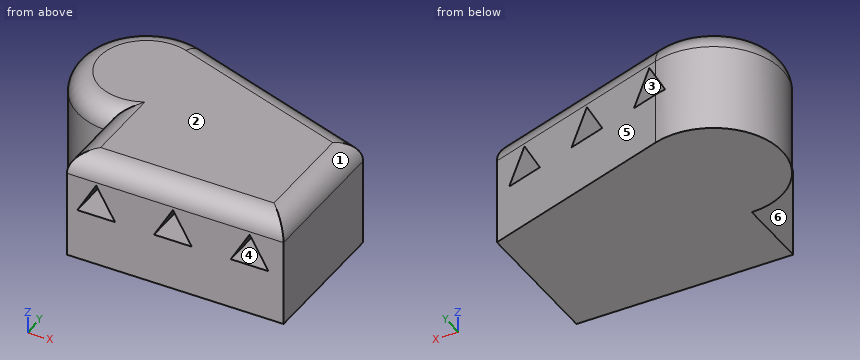
from build123d import *

# Parameters (mm, degrees)
F1_DEPTH = 25
F4_DEPTH = 25
F5_DEPTH = 23.7095438224
F6_R     = 5


# Not quite as in the source:
# - the program builds the solid bodies; features that only make, move or delete a surface that nothing else refers to are left out


with BuildPart() as f1:
    # F0 (on Top) → F1 (new body)
    with BuildSketch(Plane.XY):
        with BuildLine():
            ThreePointArc((-24.4463197887, 8.4633977604), (-29.1204506303, 19.7477478306), (-17.8361005601, 15.073616989))
            Line((-17.8361005601, 15.073616989), (-8.6304908186, 15.073616989))
            ThreePointArc((-8.6304908186, 15.073616989), (-11.6154192696, 24.3206942504), (-19.4435108685, 30.0773614855))
            ThreePointArc((-19.4435108685, 30.0773614855), (-40.0578075922, 17.607762717), (-24.4463197887, -0.7422119811))
            Line((-24.4463197887, -0.7422119811), (-24.4463197887, 8.4633977604))
        make_face()
        with BuildLine():
            Line((-17.8361005601, 15.073616989), (-24.4463197887, 15.073616989))
            Line((-24.4463197887, 15.073616989), (-24.4463197887, 8.4633977604))
            ThreePointArc((-24.4463197887, 8.4633977604), (-19.772188947, 10.3994861473), (-17.8361005601, 15.073616989))
        make_face()
        with BuildLine():
            Line((-24.4463197887, 8.4633977604), (-24.4463197887, 15.073616989))
            Line((-24.4463197887, 15.073616989), (-17.8361005601, 15.073616989))
            ThreePointArc((-17.8361005601, 15.073616989), (-29.1204506303, 19.7477478306), (-24.4463197887, 8.4633977604))
        make_face()
        with BuildLine():
            ThreePointArc((-19.4435108685, 30.0773614855), (-11.6154192696, 24.3206942504), (-8.6304908186, 15.073616989))
            Line((-8.6304908186, 15.073616989), (25.5536802113, 15.073616989))
            Line((25.5536802113, 15.073616989), (-19.4435108685, 30.0773614855))
        make_face()
        with BuildLine():
            Line((25.5536802113, 15.073616989), (-8.6304908186, 15.073616989))
            ThreePointArc((-8.6304908186, 15.073616989), (-13.2628398739, 3.8901370741), (-24.4463197887, -0.7422119811))
            Line((-24.4463197887, -0.7422119811), (-24.4463197887, -17.8190978634))
            Line((-24.4463197887, -17.8190978634), (25.5536802113, -17.8190978634))
            Line((25.5536802113, -17.8190978634), (25.5536802113, 15.073616989))
        make_face()
        with BuildLine():
            Line((-8.6304908186, 15.073616989), (-17.8361005601, 15.073616989))
            ThreePointArc((-17.8361005601, 15.073616989), (-19.772188947, 10.3994861473), (-24.4463197887, 8.4633977604))
            Line((-24.4463197887, 8.4633977604), (-24.4463197887, -0.7422119811))
            ThreePointArc((-24.4463197887, -0.7422119811), (-13.2628398739, 3.8901370741), (-8.6304908186, 15.073616989))
        make_face()
    extrude(amount=F1_DEPTH)

    # F3 (on face) → F4 (cut)
    with BuildSketch(Plane.XZ.offset(17.8190978634)):
        Polygon((-22.0338956294, 11.7883440107), (-13.3311382654, 11.7883440107), (-17.6825169474, 19.3251529709), align=None)
        Polygon((4.3688617346, 11.7883440107), (0.0174830526, 19.3251529709), (-4.3338956294, 11.7883440107), align=None)
        Polygon((22.0688617346, 11.7883440107), (17.7174830526, 19.3251529709), (13.3661043706, 11.7883440107), align=None)
    extrude(amount=-F4_DEPTH, mode=Mode.SUBTRACT)

    # F5 (cut, through all): faces of the model
    f5_faces = [f1.faces().sort_by_distance(p)[0] for p in [
        (-17.6825169474, 7.1809021366, 14.3006136641),
        (0.0174830526, 7.1809021366, 14.3006136641),
        (17.7174830526, 7.1809021366, 14.3006136641),
    ]]
    extrude(f5_faces, amount=-F5_DEPTH, mode=Mode.SUBTRACT)

    # F6
    f6_edges = [f1.edges().sort_by_distance(p)[0] for p in [
        (-40.057808, 17.607763, 25),
        (-24.44632, -9.280655, 25),
        (0.55368, -17.819098, 25),
        (25.55368, -1.37274, 25),
        (3.055085, 22.575489, 25),
    ]]
    fillet(f6_edges, radius=F6_R)


solid = f1.part
CAD build for the part. Positions are in the model's coordinates, mm. Face numbers are marked on the shaded views. A direction names the side the tool comes from. Round coordinates to 2 decimals unless told otherwise and drop trailing zeros. Write each loop counter-clockwise with the first axis right and the second up, starting at its lowest first coordinate (ties: lowest second). Pieces come first, ordered by that corner, then holes.
(1) Slice it at D-D, the plane y = 17. Count the separate pieces of the cut face and the enclosed holes in it, and give its area (3 significant figures).
(2) Slice it at A-A, the plane y = -10. Write the cut outline in (x, z).
(3) Slice it at B-B, the plane z = 17.5. Write the cut outline in (x, y), and give its area (3 significant figures).
(4) Drop flat-ended pins along their axis: P1, Ø1.5, axis at y = -4.5, z = 20.5, coming from the -X side; P2, Ø12, axis at y = 0, z = 22, coming from the -X side; P3, Ø6, axis at x = 11.5, y = 25, coming from the -Z side. Give the stop position or say it passes through.
(5) Slice it at C-C, the plane z = 11. Write the cut outline in (x, y).
(6) Probe line 1 along X through (y, z) = (-9.5, 13.25); line 2 along X through (y, z) = (17, 15.25); line 3 along X through (y, z) = (-5.5, 13.5). List the from-to ranges inside material, lowest first.
(7) Mould opens along X. For the marked faces 1, 2 and 3 say: pulls with the +X half, pulls with the -X half, needs draft (parallel to the pull), parting line crosses it, or undercut.
(8) 3-axis set-ups, long thin cutter, end or side, ignore diameter. For the marked faces 4, 5 and 6: which of +Z, -Z, +X, -X, +Y, -Y reach the whole face in a straight line?
From the geometry:
1. separate pieces: 1
1. enclosed holes: 2
1. area: 1,380 mm2
2. outline: (-24.45, 0) - (25.55, 0) - (25.55, 20) arc R5 ccw to (20.55, 25) - (-19.45, 25) arc R5 ccw to (-24.45, 20) - close; hole (-22.03, 11.79) - (-13.33, 11.79) - (-17.68, 19.33) - close; hole (-4.33, 11.79) - (4.37, 11.79) - (0.02, 19.33) - close; hole (13.37, 11.79) - (22.07, 11.79) - (17.72, 19.33) - close
3. outline: (-24.45, -17.82) - (-18.74, -17.82) - (-18.74, 29.84) - (-19.44, 30.08) arc R15.82 ccw (long way) to (-24.45, -0.74) - close; (-16.63, -17.82) - (-1.04, -17.82) - (-1.04, 23.94) - (-16.63, 29.14) - close; (1.07, -17.82) - (16.66, -17.82) - (16.66, 18.04) - (1.07, 23.24) - close; (18.77, -17.82) - (25.55, -17.82) - (25.55, 15.07) - (18.77, 17.34) - close
3. area: 2,190 mm2
4. P1: stops at x = -24.45
4. P2: stops at x = -37.24
4. P3: passes through
5. outline: (-24.45, -17.82) - (25.55, -17.82) - (25.55, 15.07) - (-19.44, 30.08) arc R15.82 ccw (long way) to (-24.45, -0.74) - close
6. line 1: x = -24.45 to -21.19, -14.18 to -3.49, 3.52 to 14.21, 21.22 to 25.55
6. line 2: x = -40.14 to -20.04, -15.33 to -2.34, 2.37 to 15.36
6. line 3: x = -24.45 to -21.05, -14.32 to -3.35, 3.38 to 14.35, 21.08 to 25.55
7. face 1: pulls with the +X half
7. face 2: needs draft
7. face 3: undercut
8. face 4: +Y, -Y
8. face 5: +Z, -Z, +X, +Y
8. face 6: +Z, -Z, -X, -Y
